Input: part model. Units: mm. Frame: model coordinates. A direction names the side the tool comes from. Round coordinates to 2 decimals unless told otherwise and drop trailing zeros. Loops run counter-clockwise (first coordinate to the right, second up) from the corner with the lowest first, then second, coordinate; pieces in that order, holes last. Notation, with made-up numbers: (-16.75, 37.5) -> (21.25, 37.5) arc R28 cw to (21.25, 59.5) -> close; hole circle Ø6 at (-30, -5.75). An arc over 180 degrees is marked (long way). Answer in a Markdown table with one row per item. Add a question column.
Q1. Section A-A, the plane x = 0. Output: boundary loops of the cut face in (y, z), and give its area (3 significant figures).
Q2. Section B-B, the plane y = -12.5. Output: boundary loops of the cut face in (x, z).
Q3. Section C-C, the plane z = -7. Output: boundary loops of the cut face in (x, y), and give its area (3 significant figures).
Q4. Section D-D, the plane x = 27. Output: boundary loops of the cut face in (y, z), and give its area (3 significant figures).
Q5. Pin query (flat end, axial travel): pin 1 (10.5 mm diameter, centred on x = -33.27, y = -10.76, fed in from +Z); pin 2 (10 mm diameter, centred on x = 20.5, y = -12, fed in from +Z); pin 3 (10.5 mm diameter, centred on x = 28.5, y = -11.5, fed in from +Z). Return the tip coordinate at first contact, or that it passes through.
Q6. Ray query, L1, parallel to Y at x = -33.5, z = 0; L2, parallel to X at y = -13.75, z = 0; L3, parallel to X at y = -9.25, z = 1. Return the intervals inside material, ascending. Write a range as from..to.
Q7. Reachability of faces 1 (the face through (28, -12, 10)), 2 (the face through (-33, -23, 9)), 3 (the face through (-33, -2, 9)), 4 (the face through (-29, -12, 10)) from +Z, -Z, +X, -X, +Y, -Y: full face, straight path, thin tool, end or side. Return the list, or none.
```python
from build123d import *

# Parameters (mm, degrees)
F0_R         = 11
F1_DEPTH     = 25
F2_R         = 4
F4_DEPTH     = 25
F3_R         = 4
F5_DEPTH     = 25
F6_S2_W      = 5
F6_S2_H      = 5
F6_T3_DEPTH  = 5
F6_T8_ANGLE  = 157.7136601513
F6_T11_DEPTH = 32.5
F6_T14_DEPTH = 27.5
F6_T17_ANGLE = 157.7136601513
F6_T20_DEPTH = 50
F6_T23_ANGLE = 78.8568300757
F6_T26_ANGLE = 78.8568300757
F6_T29_DEPTH = 27.1160389937
F6_T32_DEPTH = 27.1160389937
F6_T35_ANGLE = 78.8568300757
F6_T38_ANGLE = 78.8568300757
F6_T41_DEPTH = 27.1160389937
F6_T44_DEPTH = 9.6160389937
F7_T1_DEPTH  = 27.5
F7_S5_W      = 5
F7_S5_H      = 5
F7_T6_DEPTH  = 5


# Not quite as in the source:
# - a fillet or chamfer that OpenCascade refuses, or shapes differently, is made with other operations: its cross-section is extruded or revolved along the edge and cut away or added


with BuildPart() as f1:
    # F0 (on Front) → F1 (new body)
    with BuildSketch(Plane.XZ):
        with BuildLine():
            Line((-40, 10), (-40, -10))
            Line((-40, -10), (40, -10))
            Line((40, -10), (40, 10))
            Line((40, 10), (25.3839610063, 10))
            ThreePointArc((25.3839610063, 10), (22.2083926988, 11.137906536), (20.4782243644, 14.0336936303))
            ThreePointArc((20.4782243644, 14.0336936303), (0, 30.8717118949), (-20.4782243644, 14.0336936303))
            ThreePointArc((-20.4782243644, 14.0336936303), (-22.2083926988, 11.137906536), (-25.3839610063, 10))
            Line((-25.3839610063, 10), (-40, 10))
        make_face()
        with Locations((0, 10)):
            Circle(F0_R, mode=Mode.SUBTRACT)
    extrude(amount=F1_DEPTH)

    # F2 (on face) → F4 (cut)
    with BuildSketch(Plane.XY.offset(10)):
        with Locations((32.6919805032, -12.5)):
            Circle(F2_R)
    extrude(amount=-F4_DEPTH, mode=Mode.SUBTRACT)

    # F3 (on face) → F5 (cut)
    with BuildSketch(Plane.XY.offset(10)):
        with Locations((-33.267121762, -10.7605047524)):
            Circle(F3_R)
    extrude(amount=-F5_DEPTH, mode=Mode.SUBTRACT)

    # F6: fillet of radius 5 on 5 edges, made by hand


with BuildPart() as f6_tool1:
    # F6_s2 → F6_t3 (new body)
    with BuildSketch(Plane.YZ.offset(35)):
        with Locations((-22.5, 7.5)):
            Rectangle(F6_S2_W, F6_S2_H)
    extrude(amount=F6_T3_DEPTH)

    # F6_s4 → F6_t5 (revolve, cut)
    with BuildSketch(Plane(origin=(35, -20, 5), x_dir=(0, 0.7071067812, -0.7071067812), z_dir=(0, -0.7071067812, -0.7071067812))):
        with BuildLine():
            ThreePointArc((0, -5), (5, 0), (0, 5))
            Line((0, 5), (0, -5))
        make_face()
    revolve(axis=Axis((35, -20, 5), (1, 0, 0)), mode=Mode.SUBTRACT)


with BuildPart() as f6_tool6:
    # F6_s7 → F6_t8 (revolve)
    with BuildSketch(Plane(origin=(-1.8961778261, 0, 9.6265007999), x_dir=(0, 1, 0), z_dir=(0.1932612739, 0, -0.9811473284))):
        with BuildLine():
            ThreePointArc((-20, 22.8043246343), (-23.5355339059, 21.3398585403), (-25, 17.8043246343))
            Line((-25, 17.8043246343), (-25, 22.8043246343))
            Line((-25, 22.8043246343), (-20, 22.8043246343))
        make_face()
    revolve(axis=Axis((0, -25, 10), (0, -1, 0)), revolution_arc=F6_T8_ANGLE)


with BuildPart() as f6_tool9:
    # F6_s10 → F6_t11 (new body)
    with BuildSketch(Plane.XZ.offset(-12.5)):
        with BuildLine():
            ThreePointArc((40, 5), (38.5355339059, 8.5355339059), (35, 10))
            Line((35, 10), (40, 10))
            Line((40, 10), (40, 5))
        make_face()
    extrude(amount=F6_T11_DEPTH)


with BuildPart() as f6_tool12:
    # F6_s13 → F6_t14 (new body)
    with BuildSketch(Plane.XY.offset(-22.5)):
        with BuildLine():
            ThreePointArc((35, -25), (38.5355339059, -23.5355339059), (40, -20))
            Line((40, -20), (40, -25))
            Line((40, -25), (35, -25))
        make_face()
    extrude(amount=F6_T14_DEPTH)


with BuildPart() as f6_tool15:
    # F6_s16 → F6_t17 (revolve)
    with BuildSketch(Plane(origin=(-1.8961778261, 0, 9.6265007999), x_dir=(0, 1, 0), z_dir=(0.1932612739, 0, -0.9811473284))):
        with BuildLine():
            ThreePointArc((-5, 22.8043246343), (-1.4644660941, 21.3398585403), (0, 17.8043246343))
            Line((0, 17.8043246343), (0, 22.8043246343))
            Line((0, 22.8043246343), (-5, 22.8043246343))
        make_face()
    revolve(axis=Axis((0, 0, 10), (0, -1, 0)), revolution_arc=F6_T17_ANGLE)


with BuildPart() as f6_tool18:
    # F6_s19 → F6_t20 (new body)
    with BuildSketch(Plane.XZ.offset(-12.5)):
        with BuildLine():
            ThreePointArc((-35, 10), (-38.5355339059, 8.5355339059), (-40, 5))
            Line((-40, 5), (-40, 10))
            Line((-40, 10), (-35, 10))
        make_face()
    extrude(amount=F6_T20_DEPTH)


with BuildPart() as f6_tool21:
    # F6_s22 → F6_t23 (revolve)
    with BuildSketch(Plane.YZ.offset(25.3839610063)):
        with BuildLine():
            ThreePointArc((0, 5), (-1.4644660941, 8.5355339059), (-5, 10))
            Line((-5, 10), (0, 10))
            Line((0, 10), (0, 5))
        make_face()
    revolve(axis=Axis((25.3839610063, 0, 15), (0, 1, 0)), revolution_arc=F6_T23_ANGLE)


with BuildPart() as f6_tool24:
    # F6_s25 → F6_t26 (revolve)
    with BuildSketch(Plane(origin=(1.8961778261, 0, 9.6265007999), x_dir=(0, 1, 0), z_dir=(0.1932612739, 0, 0.9811473284))):
        with BuildLine():
            ThreePointArc((-5, 22.8043246343), (-1.4644660941, 21.3398585403), (0, 17.8043246343))
            Line((0, 17.8043246343), (0, 22.8043246343))
            Line((0, 22.8043246343), (-5, 22.8043246343))
        make_face()
    revolve(axis=Axis((-25.3839610063, 0, 15), (0, 1, 0)), revolution_arc=F6_T26_ANGLE)


with BuildPart() as f6_tool27:
    # F6_s28 → F6_t29 (new body)
    with BuildSketch(Plane.YZ.offset(-25.3839610063)):
        with BuildLine():
            ThreePointArc((-5, 10), (-1.4644660941, 8.5355339059), (0, 5))
            Line((0, 5), (0, 10))
            Line((0, 10), (-5, 10))
        make_face()
    extrude(amount=-F6_T29_DEPTH)


with BuildPart() as f6_tool30:
    # F6_s31 → F6_t32 (new body)
    with BuildSketch(Plane.YZ.offset(52.5)):
        with BuildLine():
            ThreePointArc((0, 5), (-1.4644660941, 8.5355339059), (-5, 10))
            Line((-5, 10), (0, 10))
            Line((0, 10), (0, 5))
        make_face()
    extrude(amount=-F6_T32_DEPTH)


with BuildPart() as f6_tool33:
    # F6_s34 → F6_t35 (revolve)
    with BuildSketch(Plane.YZ.offset(25.3839610063)):
        with BuildLine():
            ThreePointArc((-25, 5), (-23.5355339059, 8.5355339059), (-20, 10))
            Line((-20, 10), (-25, 10))
            Line((-25, 10), (-25, 5))
        make_face()
    revolve(axis=Axis((25.3839610063, -25, 15), (0, 1, 0)), revolution_arc=F6_T35_ANGLE)


with BuildPart() as f6_tool36:
    # F6_s37 → F6_t38 (revolve)
    with BuildSketch(Plane(origin=(1.8961778261, 0, 9.6265007999), x_dir=(0, 1, 0), z_dir=(0.1932612739, 0, 0.9811473284))):
        with BuildLine():
            ThreePointArc((-20, 22.8043246343), (-23.5355339059, 21.3398585403), (-25, 17.8043246343))
            Line((-25, 17.8043246343), (-25, 22.8043246343))
            Line((-25, 22.8043246343), (-20, 22.8043246343))
        make_face()
    revolve(axis=Axis((-25.3839610063, -25, 15), (0, 1, 0)), revolution_arc=F6_T38_ANGLE)


with BuildPart() as f6_tool39:
    # F6_s40 → F6_t41 (new body)
    with BuildSketch(Plane.YZ.offset(-25.3839610063)):
        with BuildLine():
            ThreePointArc((-20, 10), (-23.5355339059, 8.5355339059), (-25, 5))
            Line((-25, 5), (-25, 10))
            Line((-25, 10), (-20, 10))
        make_face()
    extrude(amount=-F6_T41_DEPTH)


with BuildPart() as f6_tool42:
    # F6_s43 → F6_t44 (new body)
    with BuildSketch(Plane.YZ.offset(35)):
        with BuildLine():
            ThreePointArc((-25, 5), (-23.5355339059, 8.5355339059), (-20, 10))
            Line((-20, 10), (-25, 10))
            Line((-25, 10), (-25, 5))
        make_face()
    extrude(amount=-F6_T44_DEPTH)


with BuildPart() as f1_1:
    add(f1.part)

    # F6_t45: cut F6_tool1, F6_tool6, F6_tool9, F6_tool12, F6_tool15, F6_tool18, F6_tool21, F6_tool24, F6_tool27, F6_tool30, F6_tool33, F6_tool36, F6_tool39, F6_tool42
    add([f6_tool1.part, f6_tool6.part, f6_tool9.part, f6_tool12.part, f6_tool15.part, f6_tool18.part, f6_tool21.part, f6_tool24.part, f6_tool27.part, f6_tool30.part, f6_tool33.part, f6_tool36.part, f6_tool39.part, f6_tool42.part], mode=Mode.SUBTRACT)

    # F7: fillet of radius 5 on 1 edges, made by hand

    # F7_s2 → F7_t1 (cut)
    with BuildSketch(Plane.XY.offset(-22.5)):
        with BuildLine():
            ThreePointArc((35, 0), (38.5355339059, -1.4644660941), (40, -5))
            Line((40, -5), (40, 0))
            Line((40, 0), (35, 0))
        make_face()
    extrude(amount=F7_T1_DEPTH, mode=Mode.SUBTRACT)


with BuildPart() as f7_tool4:
    # F7_s5 → F7_t6 (new body)
    with BuildSketch(Plane.XZ.offset(5)):
        with Locations((37.5, 7.5)):
            Rectangle(F7_S5_W, F7_S5_H)
    extrude(amount=-F7_T6_DEPTH)

    # F7_s7 → F7_t8 (revolve, cut)
    with BuildSketch(Plane(origin=(35, -5, 5), x_dir=(-0.7071067812, 0, -0.7071067812), z_dir=(0.7071067812, 0, -0.7071067812))):
        with BuildLine():
            ThreePointArc((0, -5), (5, 0), (0, 5))
            Line((0, 5), (0, -5))
        make_face()
    revolve(axis=Axis((35, -5, 5), (0, 1, 0)), mode=Mode.SUBTRACT)


with BuildPart() as f1_2:
    add(f1_1.part)

    # F7_t3: cut F7_tool4
    add(f7_tool4.part, mode=Mode.SUBTRACT)


solid = f1_2.part
```
Answer block:
| question | item | result |
|---|---|---|
| 1 | outline | (-25, -10) -> (0, -10) -> (0, -1) -> (-25, -1) -> close; (-25, 21) -> (0, 21) -> (0, 25.87) arc R5 ccw to (-5, 30.87) -> (-20, 30.87) arc R5 ccw to (-25, 25.87) -> close |
| 1 | area | 461 mm^2 |
| 2 | outline | (-40, -10) -> (-36.87, -10) -> (-36.87, 9.64) arc R5 ccw to (-40, 5) -> close; (-29.67, -10) -> (28.69, -10) -> (28.69, 10) -> (25.38, 10) arc R5 cw to (20.48, 14.03) arc R20.87 ccw to (-20.48, 14.03) arc R5 cw to (-25.38, 10) -> (-29.67, 10) -> close; (36.69, -10) -> (40, -10) -> (40, 5) arc R5 ccw to (36.69, 9.71) -> close; hole circle Ø22 at (0, 10) |
| 3 | outline | (-40, -25) -> (35, -25) arc R5 ccw to (40, -20) -> (40, -5) arc R5 ccw to (35, 0) -> (-40, 0) -> close; hole circle Ø8 at (-33.27, -10.76); hole circle Ø8 at (32.69, -12.5) |
| 3 | area | 1,890 mm^2 |
| 4 | outline | (-25, -10) -> (0, -10) -> (0, 5) arc R5 ccw to (-5, 10) -> (-20, 10) arc R5 ccw to (-25, 5) -> close |
| 4 | area | 489 mm^2 |
| 5 | pin 1 | z = 10 |
| 5 | pin 2 | z = 23.98 |
| 5 | pin 3 | z = 10.48 |
| 6 | L1 | -25..-14.75, -6.77..0 |
| 6 | L2 | -40..-35.92, -30.61..-4.58, 4.58..28.89, 36.49..40 |
| 6 | L3 | -40..-36.97, -29.56..-6.32, 6.32..30.36, 35.02..40 |
| 7 | face 1 | +Z, +X, +Y, -Y |
| 7 | face 2 | +Z, -X, -Y |
| 7 | face 3 | +Z, -X, +Y |
| 7 | face 4 | +Z, -X, +Y, -Y |
